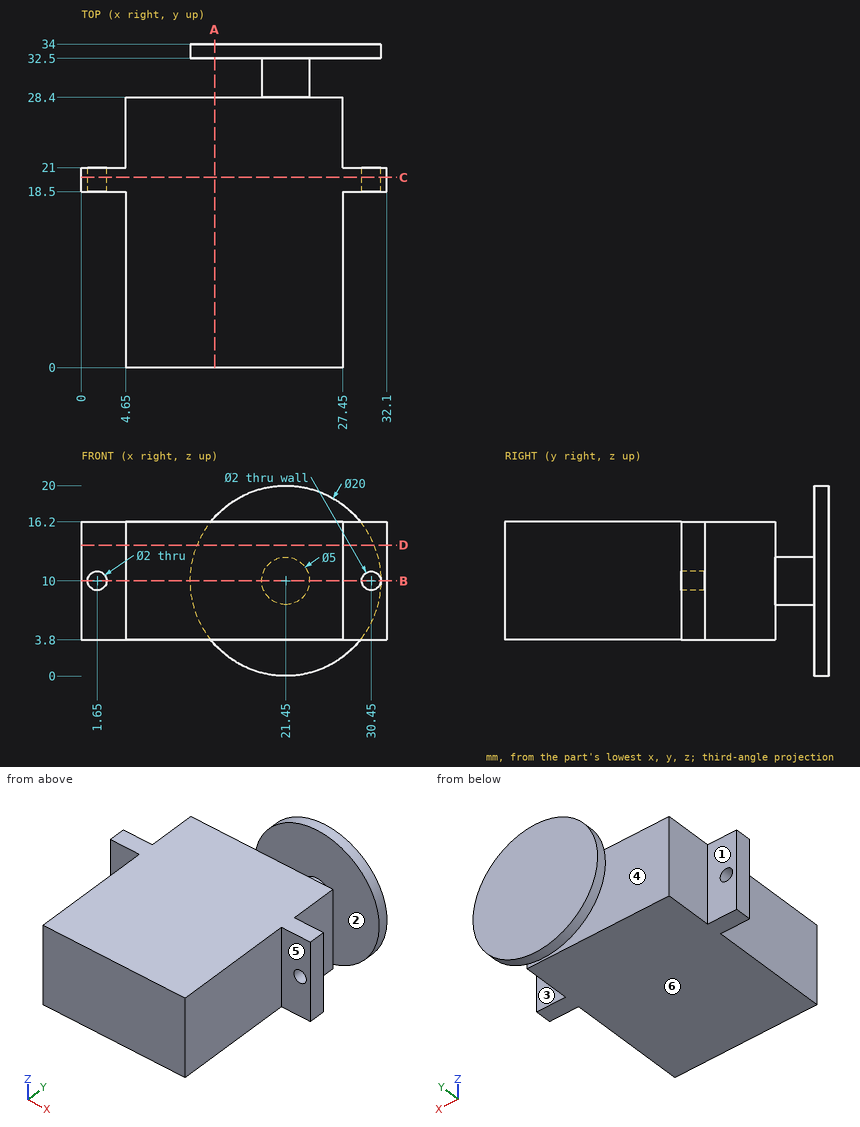
The drawing under review shows one solid part. Ordinate dimensions are in mm from its lowest x, y, z. A direction names the side the tool comes from. Coordinates: 2 decimals unless noted, no trailing zeros. Loops run counter-clockwise (first coordinate to the right, second up) from the corner with the lowest first, then second, coordinate; pieces in that order, holes last. Notation, with made-up numbers: (55.25, 62.5) - (105.25, 62.5) arc R26 cw to (105.25, 96.5) - close; hole circle Ø8 at (46, -2.5). An arc over 180 degrees is marked (long way). Use CSV: the item, a comma, the result in double quotes. Start each with the question number.
1. Clearance check with flat-ended pins moving along their axes: pin 1 (6 mm diameter, centred on y = 9.5, z = 3.5, fed in from +X); pin 2 (1.5 mm diameter, centred on x = 11.5, y = 20, fed in from +Z); pin 3 (2 mm diameter, centred on x = 18, y = 7.5, fed in from -Z); pin 4 (1.8 mm diameter, centred on x = 1.65, z = 10, fed in from +Y). State where each tip first meets the part, or that it passes through.
2. Mouldability with a two-part tool opening along Y and no side actions: class the marked faces 4, 5 and 6 as released by +Y, released by -Y, zero draft, split by the parting line, or undercut.
3. Add section C-C on y = 20. Give the boundary of the cut face in (x, z).
4. For the marked faces 1, 2 and 3, list the 3-axis set-ups (+Z, -Z, +X, -X, +Y, -Y) from which the entire face can be reached by the end or side of a thin tool; tool diameter is ignored.
5. To check wall thickness, follow probe 1 along X at (y, z) = (19.1, 10); probe 2 along Y at (x, z) = (17.5, 4); probe 3 along X at (y, z) = (14.5, 4.5). State the ranges of each line that lie inside material, in increasing order.
6. Add section D-D on z = 13.75. Give the boundary of the cut face in (x, y), plus the area to 3 significant figures.
7. Add section A-A on x = 14. Give the boundary of the cut face in (y, z).
8. Add section B-B on z = 10. Give the boundary of the cut face in (x, y), plus the area to 3 significant figures.
Resolved:
1,pin 1,"x = 27.45"
1,pin 2,"z = 16.2"
1,pin 3,"z = 3.8"
1,pin 4,"through"
2,face 4,"undercut"
2,face 5,"released by -Y"
2,face 6,"zero draft"
3,outline,"(0, 3.8) - (32.1, 3.8) - (32.1, 16.2) - (0, 16.2) - close; hole circle Ø2 at (1.65, 10); hole circle Ø2 at (30.45, 10)"
4,face 1,"+Z, -Z, -X, +Y"
4,face 2,"none"
4,face 3,"+Z, -Z, +X"
5,probe 1,"0 to 0.65, 2.65 to 29.45, 31.45 to 32.1"
5,probe 2,"0 to 28.4, 32.5 to 34"
5,probe 3,"4.65 to 27.45"
6,outline,"(0, 18.5) - (4.65, 18.5) - (4.65, 0) - (27.45, 0) - (27.45, 18.5) - (32.1, 18.5) - (32.1, 21) - (27.45, 21) - (27.45, 28.4) - (4.65, 28.4) - (4.65, 21) - (0, 21) - close; (12.18, 32.5) - (30.72, 32.5) - (30.72, 34) - (12.18, 34) - close"
6,area,"699 mm2"
7,outline,"(0, 3.8) - (28.4, 3.8) - (28.4, 16.2) - (0, 16.2) - close; (32.5, 3.33) - (34, 3.33) - (34, 16.67) - (32.5, 16.67) - close"
8,outline,"(0, 18.5) - (0.65, 18.5) - (0.65, 21) - (0, 21) - close; (2.65, 18.5) - (4.65, 18.5) - (4.65, 0) - (27.45, 0) - (27.45, 18.5) - (29.45, 18.5) - (29.45, 21) - (27.45, 21) - (27.45, 28.4) - (23.95, 28.4) - (23.95, 32.5) - (31.45, 32.5) - (31.45, 34) - (11.45, 34) - (11.45, 32.5) - (18.95, 32.5) - (18.95, 28.4) - (4.65, 28.4) - (4.65, 21) - (2.65, 21) - close; (31.45, 18.5) - (32.1, 18.5) - (32.1, 21) - (31.45, 21) - close"
8,area,"711 mm2"
